For this review, take the finished solid that the model builds, in its own axes (mm). A direction names the side the tool comes from. Coordinates: 2 decimals unless noted, no trailing zeros. Order: outer loops, then holes, each group sorted by start corner. A loop starts at its lowest first (then second) coordinate and runs counter-clockwise, first axis right, second up. Notation, with made-up numbers: (-30.75, 10.25) -> (-24.75, 10.25) arc R17 ccw to (-24.75, 19.25) -> close; hole circle Ø8 at (41, 55). An arc over 180 degrees is marked (long way). Answer as a JSON object with one key per item and string values. Group by question number.
1) Machinability: for faces 1 (the cylindrical face through (27.43, 2.59, 1.48)), 2 (the cylindrical face through (28.5, 0.07, 1.48)), 3 (the flat face through (15, -2.5, 1)), which of the approach directions +Z, -Z, +X, -X, +Y, -Y give a long, thin tool a straight path to every point of the face, cutting with its end or side? Answer none if there is none.
2) For pin 1 (1.5 mm diameter, centred on x = 22.5, z = 1, fed in from -Y); pin 2 (4 mm diameter, centred on x = 30, y = 0, fed in from +Z), all flat-tipped, find the tip position at first contact; note any pin that passes through.
3) Draft analysis for pull direction X (two halves, no side actions). For faces 4 (the flat face through (15, 0, 0)), 5 (the flat face through (15, 2.5, 1)), 6 (the cylindrical face through (27.449, -2.596, 1.479)), state which applies: +X half, -X half, draft (parallel to the pull), parting line (faces both ways), or undercut.
4) Add section C-C, the plane z = 0.9. Write out the cut boundary in (x, y), then the cut area to 3 significant figures.
5) Add section D-D, the plane x = 21.5. Write out the cut boundary in (y, z).
6) Wall thickness on L1, parallel to Y at x = 0, z = 1.1; L2, parallel to X at y = 1, z = 0.4; L3, parallel to X at y = -0.5, z = 2.1: over which ranges is each line inside the solid? List them lowest first.
7) Add section A-A, the plane x = 30. Write out the cut boundary in (y, z).
8) Add section B-B, the plane y = 0. Write out the cut boundary in (x, z), then the cut area to 3 significant figures.
from build123d import *

# Parameters (mm, degrees)
SKETCH_1_R      = 1.5
EXTRUDE_1_DEPTH = 3


with BuildPart() as part:
    # 草图1 → 凸台-拉伸1 (new body)
    with BuildSketch(Plane.XY):
        with BuildLine():
            Line((3.16227766, 2.5), (26.83772234, 2.5))
            ThreePointArc((26.83772234, 2.5), (27.440745029, 2.593074822), (27.987641489, 2.863636364))
            ThreePointArc((27.987641489, 2.863636364), (33.5, 0), (27.987641489, -2.863636364))
            ThreePointArc((27.987641489, -2.863636364), (27.440745029, -2.593074822), (26.83772234, -2.5))
            Line((26.83772234, -2.5), (3.16227766, -2.5))
            ThreePointArc((3.16227766, -2.5), (2.559254971, -2.593074822), (2.012358511, -2.863636364))
            ThreePointArc((2.012358511, -2.863636364), (-3.5, 0), (2.012358511, 2.863636364))
            ThreePointArc((2.012358511, 2.863636364), (2.559254971, 2.593074822), (3.16227766, 2.5))
        make_face()
        Circle(SKETCH_1_R, mode=Mode.SUBTRACT)
        with Locations((30, 0)):
            Circle(SKETCH_1_R, mode=Mode.SUBTRACT)
    extrude(amount=EXTRUDE_1_DEPTH)


solid = part.part
Output values:
{
 "1": {"face 1": "+Z, -Z, +Y", "face 2": "+Z, -Z", "face 3": "+Z, -Z, -Y"},
 "2": {"pin 1": "stops at y = -2.5", "pin 2": "stops at z = 3"},
 "3": {"face 4": "draft", "face 5": "undercut", "face 6": "undercut"},
 "4": {"outline": "(2.01, -2.86) arc R2 cw to (3.16, -2.5) -> (26.84, -2.5) arc R2 cw to (27.99, -2.86) arc R3.5 ccw (long way) to (27.99, 2.86) arc R2 cw to (26.84, 2.5) -> (3.16, 2.5) arc R2 cw to (2.01, 2.86) arc R3.5 ccw (long way) to start; hole circle Ø3 at (0, 0); hole circle Ø3 at (30, 0)", "area": "181 mm²"},
 "5": {"outline": "(-2.5, 0) -> (2.5, 0) -> (2.5, 3) -> (-2.5, 3) -> close"},
 "6": {"L1": "y = -3.5 to -1.5, 1.5 to 3.5", "L2": "x = -3.35 to -1.12, 1.12 to 28.88, 31.12 to 33.35", "L3": "x = -3.46 to -1.41, 1.41 to 28.59, 31.41 to 33.46"},
 "7": {"outline": "(-3.5, 0) -> (-1.5, 0) -> (-1.5, 3) -> (-3.5, 3) -> close; (1.5, 0) -> (3.5, 0) -> (3.5, 3) -> (1.5, 3) -> close"},
 "8": {"outline": "(-3.5, 0) -> (-1.5, 0) -> (-1.5, 3) -> (-3.5, 3) -> close; (1.5, 0) -> (28.5, 0) -> (28.5, 3) -> (1.5, 3) -> close; (31.5, 0) -> (33.5, 0) -> (33.5, 3) -> (31.5, 3) -> close", "area": "93.0 mm²"}
}
